Geometry check sheet. Reference: drawing and pictorial views, mm from the part's lowest x, y, z. A direction names the side the tool comes from. Coordinates: 2 decimals unless noted, no trailing zeros. Write each loop counter-clockwise with the first axis right and the second up, starting at its lowest first coordinate (ties: lowest second). Pieces come first, ordered by that corner, then holes. Notation, with made-up numbers: (-10, -12.5) - (-1, -12.5) arc R15 cw to (-1, -3.5) - close; hole circle Ø2 at (-12.75, 5). An arc over 180 degrees is marked (long way). Use one line per item in the form item = value. Start each with the question number.
(1) Sectioned sample at D-D (y = 5.75). Record the cut outline in (x, z).
(2) Material ranges on line 1 (X direction, y = 5.5, z = 30); line 2 (X direction, y = 7, z = 4.5); line 3 (Z direction, x = 28, y = 17), recorded low to high. Write a range as [from, to].
(3) Sectioned sample at B-B (x = 5.5). Record the cut outline in (y, z) (1 decimal).
(4) Mould release check, pull along Z, two halves, no side actions. Record for the marked faces 4, 5 and 6: released by +Z, released by -Z, zero draft, split by the parting line, or undercut.
(5) Sectioned sample at A-A (y = 17). Record the cut outline in (x, z).
(6) Sectioned sample at C-C (z = 30). Record the cut outline in (x, y), and give its area (3 significant figures).
(7) Gauge pin test, flat ends, axial feed: pin 1 Ø1 at (x, y) = (15, 17) entering from +Z; pin 2 Ø9 at (x, z) = (15, 7) entering from +Y (1 decimal); pin 3 Ø3.5 at (x, z) = (11, 29) entering from +Y (1 decimal). Record the tip position at first contact, or that the pin passes through.
(8) Tool access check on the marked faces 1, 2 and 3. Record the directions out of +Z, -Z, +X, -X, +Y, -Y that give a thin tool (end or side, any length) a straight path to the whole face; none if there is none.
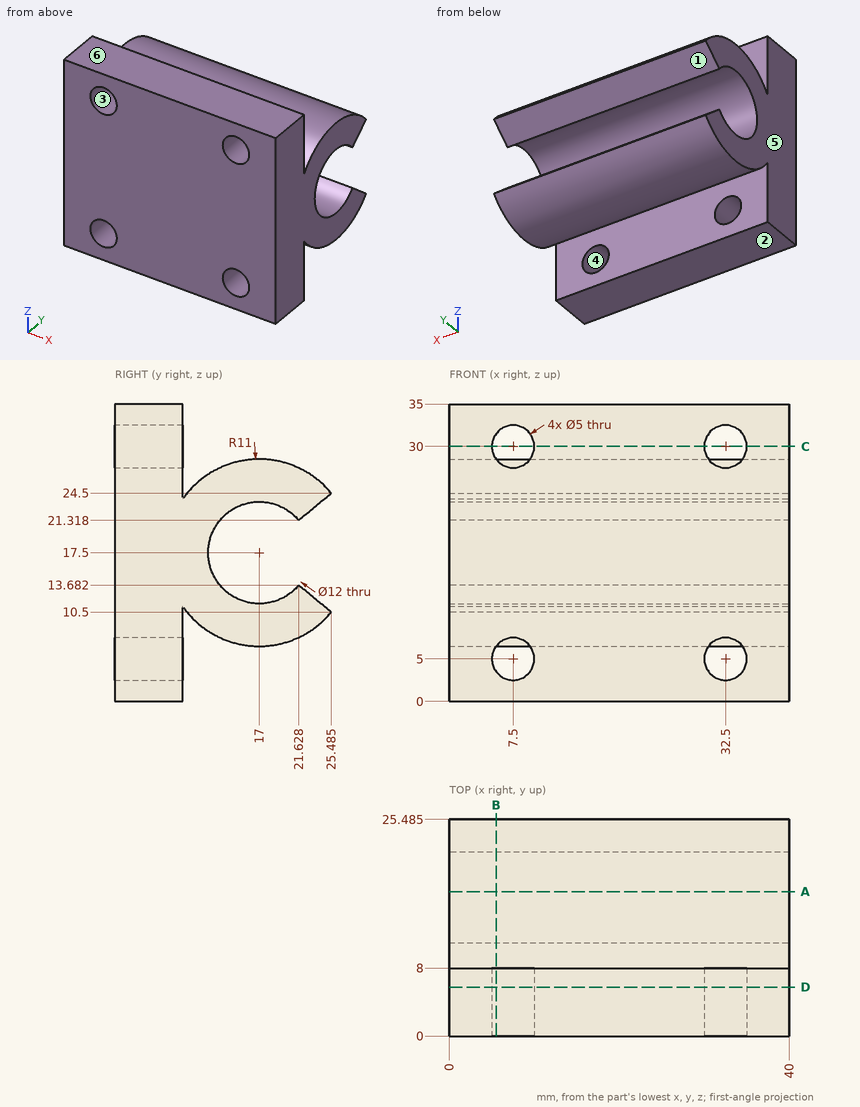
Answers below:
q1.outline = (0, 0) - (40, 0) - (40, 35) - (0, 35) - close; hole circle Ø5 at (7.5, 5); hole circle Ø5 at (7.5, 30); hole circle Ø5 at (32.5, 5); hole circle Ø5 at (32.5, 30)
q2.line_1 = [0, 5], [10, 30], [35, 40]
q2.line_2 = [0, 5.05], [9.95, 30.05], [34.95, 40]
q2.line_3 = [6.5, 11.5], [23.5, 28.5]
q3.outline = (0, 0) - (8, 0) - (8, 3.5) - (0, 3.5) - close; (0, 6.5) - (8, 6.5) - (8, 11.2) arc R11 ccw to (25.5, 10.5) - (21.6, 13.7) arc R6 cw (long way) to (21.6, 21.3) - (25.5, 24.5) arc R11 ccw to (8, 23.8) - (8, 28.5) - (0, 28.5) - close; (0, 31.5) - (8, 31.5) - (8, 35) - (0, 35) - close
q4.face_4 = undercut
q4.face_5 = zero draft
q4.face_6 = released by +Z
q5.outline = (0, 6.5) - (40, 6.5) - (40, 11.5) - (0, 11.5) - close; (0, 23.5) - (40, 23.5) - (40, 28.5) - (0, 28.5) - close
q6.outline = (0, 0) - (5, 0) - (5, 8) - (0, 8) - close; (10, 0) - (30, 0) - (30, 8) - (10, 8) - close; (35, 0) - (40, 0) - (40, 8) - (35, 8) - close
q6.area = 240 mm2
q7.pin_1 = 28.5
q7.pin_2 = 25.5
q7.pin_3 = 22.1
q8.face_1 = +X, -X, +Y
q8.face_2 = -Z, +X, -X, +Y, -Y
q8.face_3 = -Y
